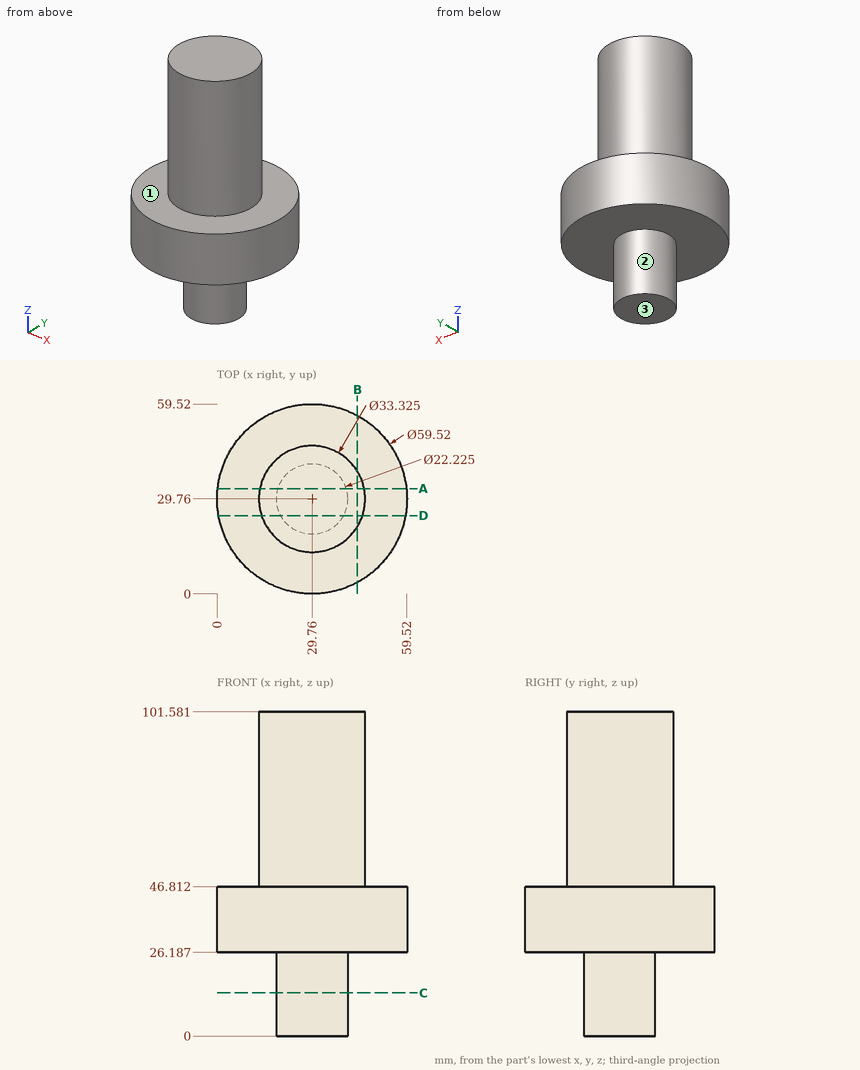
Input: dimensioned drawing with shaded views. Units: mm. Origin: part minimum x, y, z. A direction names the side the tool comes from. Give positions to 0.01 mm unless a question says otherwise; leave off trailing zeros. Order: outer loops, then holes, each group sorted by start corner. A loop starts at its lowest first (then second) coordinate and runs counter-clockwise, first axis right, second up.
(1) Material intervals for line 1 along Z through (x, y) = (11, 33); line 2 along Y through (x, z) = (30.5, 14.5); line 3 along Z through (x, y) = (30, 42.5), sorted ascending.
(2) Contact query for flat-ended pins moving along their axis: P1, Ø10, axis at x = 15.5, z = 76, coming from the -Y side; P2, Ø1, axis at x = 42.5, z = 54, coming from the -Y side (1 decimal); P3, Ø1.5, axis at y = 8.5, z = 38.5, coming from the +X side (1 decimal). Output: stop coordinate, or through.
(3) Access query for the marked faces 1, 2 and 3. Directions: +Z, -Z, +X, -X, +Y, -Y. A direction counts if a zero-diameter tool reaches every point of the face in a straight line with its end or side. Return the directions, or none.
(4) Section query D-D (y = 24.5). Return the cut outline in (x, z).
(5) Section query A-A (y = 33). Return the cut outline in (x, z) (1 decimal).
(6) Section query B-B (x = 44). Return the cut outline in (y, z).
(7) Section query C-C (z = 13.5). Return the cut outline in (x, y) (1 decimal), plus the area to 3 significant figures.
Outcome:
1. line 1: z = 26.19 to 46.81
1. line 2: y = 18.67 to 40.85
1. line 3: z = 26.19 to 101.58
2. P1: stops at y = 15.91
2. P2: stops at y = 18.5
2. P3: stops at x = 51.3
3. face 1: +Z
3. face 2: -Z
3. face 3: -Z, +X, -X, +Y, -Y
4. outline: (0.47, 26.19) - (19.97, 26.19) - (19.97, 0) - (39.55, 0) - (39.55, 26.19) - (59.05, 26.19) - (59.05, 46.81) - (45.57, 46.81) - (45.57, 101.58) - (13.95, 101.58) - (13.95, 46.81) - (0.47, 46.81) - close
5. outline: (0.2, 26.2) - (19.1, 26.2) - (19.1, 0) - (40.4, 0) - (40.4, 26.2) - (59.3, 26.2) - (59.3, 46.8) - (46.1, 46.8) - (46.1, 101.6) - (13.4, 101.6) - (13.4, 46.8) - (0.2, 46.8) - close
6. outline: (3.63, 26.19) - (55.89, 26.19) - (55.89, 46.81) - (38.41, 46.81) - (38.41, 101.58) - (21.11, 101.58) - (21.11, 46.81) - (3.63, 46.81) - close
7. outline: circle Ø22.2 at (29.8, 29.8)
7. area: 388 mm2
